Source: CAD feature listing. Evaluate the final solid. Frame: model axes, mm. A direction names the side the tool comes from. Round coordinates to 2 decimals unless told otherwise and drop trailing zeros. Loops run counter-clockwise (first coordinate to the right, second up) from the corner with the lowest first, then second, coordinate; pieces in that order, holes last. Notation, with made-up numbers: (49.25, 89.25) - (88.25, 89.25) arc R9 ccw to (88.25, 99.25) - close; hole circle Ø6 at (76.5, 66.5). An arc over 180 degrees is marked (long way). One line per question, with ' | ' between items. Start each with the question number.
1. Cut plane B-B (y = 0.4). Return loops of the section in (x, z).
2. Cut plane A-A (x = 0). Return loops of the section in (y, z).
3. Ray query, line 1 (Z direction, x = -0.5, y = 1.15); line 2 (X direction, y = 0.9, z = 8.5); line 3 (Z direction, x = -4, y = 0.95). Return the intervals inside material, ascending.
4. Cut plane C-C (z = -8.5). Return loops of the section in (x, y).
5. Access query for faces 1 (the cylindrical face through (3.035, 0.76, 4.051)), 2 (the flat face through (2.75, 1, -8)), 3 (the flat face through (-12, 1, -3.75)), 4 (the flat face through (-2.75, 1, 8)). Directions: +Z, -Z, +X, -X, +Y, -Y. A direction counts if a zero-diameter tool reaches every point of the face in a straight line with its end or side. Return the directions, or none.
6. Pin query (flat end, axial travel): pin 1 (1.4 mm diameter, centred on x = 0, z = -11.21, fed in from -Y); pin 2 (0.8 mm diameter, centred on x = 9, y = 0.5, fed in from +Z). Return the tip coordinate at first contact, or that it passes through.
7. Mould query, pull axis X, two halves, no side actions, for faces 5 (the flat face through (9, 1, 3.75)), 6 (the cylindrical face through (0.06, 0.74, -13.957)), 7 (the cylindrical face through (0.36, 0.76, 12.35)). Classes: pulls with the +X half, pulls with the -X half, needs draft (parallel to the pull), parting line crosses it, or undercut.
```python
from build123d import *

# Parameters (mm, degrees)
SKETCH1_W            = 5.5
SKETCH1_H            = 2
SKETCH1_R            = 1.25
SKETCH1_H_2          = 0.125
SKETCH1_H_3          = 3.25
SKETCH1_H_4          = 7.5
SKETCH1_W_2          = 15.49
SKETCH1_W_3          = 2
SKETCH1_W_4          = 8.01
BOSS_EXTRUDE1_DEPTH  = 1.5
M2_CLEARANCE_HOLE1_D = 2.4
FILLET1_R            = 1


with BuildPart() as part:
    # Sketch1 → Boss-Extrude1 (new body)
    # profile 1 of 16: a face of its own
    with BuildSketch(Plane(origin=(0, 0, 0), x_dir=(1, 0, 0), z_dir=(0, 1, 0))):
        with Locations((0, 8)):
            Rectangle(SKETCH1_W, SKETCH1_H)
    # profile 2 of 16: a face of its own
    with BuildSketch(Plane(origin=(0, 0, 0), x_dir=(1, 0, 0), z_dir=(0, 1, 0))):
        with BuildLine():
            Line((2.75, 9.125), (2.75, 11.2072))
            ThreePointArc((2.75, 11.2072), (0, 13.9572), (-2.75, 11.2072))
            Line((-2.75, 11.2072), (-2.75, 9.125))
            Line((-2.75, 9.125), (2.75, 9.125))
        make_face()
        with Locations((0, 11.2072)):
            Circle(SKETCH1_R, mode=Mode.SUBTRACT)
    # profile 3 of 16: a face of its own
    with BuildSketch(Plane(origin=(0, 0, 0), x_dir=(1, 0, 0), z_dir=(0, 1, 0))):
        with Locations((0, 11.2072)):
            Circle(SKETCH1_R)
    # profile 4 of 16: a face of its own
    with BuildSketch(Plane(origin=(0, 0, 0), x_dir=(1, 0, 0), z_dir=(0, 1, 0))):
        with Locations((0, 9.0625)):
            Rectangle(SKETCH1_W, SKETCH1_H_2)
    # profile 5 of 16: a face of its own
    with BuildSketch(Plane(origin=(0, 0, 0), x_dir=(1, 0, 0), z_dir=(0, 1, 0))):
        with Locations((0, 5.375)):
            Rectangle(SKETCH1_W, SKETCH1_H_3)
    # profile 6 of 16: a face of its own
    with BuildSketch(Plane(origin=(0, 0, 0), x_dir=(1, 0, 0), z_dir=(0, 1, 0))):
        Rectangle(SKETCH1_W, SKETCH1_H_4)
    # profile 7 of 16: a face of its own
    with BuildSketch(Plane(origin=(0, 0, 0), x_dir=(1, 0, 0), z_dir=(0, 1, 0))):
        with Locations((0, -5.375)):
            Rectangle(SKETCH1_W, SKETCH1_H_3)
    # profile 8 of 16: a face of its own
    with BuildSketch(Plane(origin=(0, 0, 0), x_dir=(1, 0, 0), z_dir=(0, 1, 0))):
        with Locations((-10.495, 0)):
            Rectangle(SKETCH1_W_2, SKETCH1_H_4)
    # profile 9 of 16: a face of its own
    with BuildSketch(Plane(origin=(0, 0, 0), x_dir=(1, 0, 0), z_dir=(0, 1, 0))):
        with Locations((-19.24, 0)):
            Rectangle(SKETCH1_W_3, SKETCH1_H_4)
    # profile 10 of 16: a face of its own
    with BuildSketch(Plane(origin=(0, 0, 0), x_dir=(1, 0, 0), z_dir=(0, 1, 0))):
        with Locations((6.755, 0)):
            Rectangle(SKETCH1_W_4, SKETCH1_H_4)
    # profile 11 of 16: a face of its own
    with BuildSketch(Plane(origin=(0, 0, 0), x_dir=(1, 0, 0), z_dir=(0, 1, 0))):
        with Locations((11.76, 0)):
            Rectangle(SKETCH1_W_3, SKETCH1_H_4)
    # profile 12 of 16: a face of its own
    with BuildSketch(Plane(origin=(0, 0, 0), x_dir=(1, 0, 0), z_dir=(0, 1, 0))):
        with Locations((13.76, 0)):
            Rectangle(SKETCH1_W_3, SKETCH1_H_4)
    # profile 13 of 16: a face of its own
    with BuildSketch(Plane(origin=(0, 0, 0), x_dir=(1, 0, 0), z_dir=(0, 1, 0))):
        with Locations((0, -8)):
            Rectangle(SKETCH1_W, SKETCH1_H)
    # profile 14 of 16: a face of its own
    with BuildSketch(Plane(origin=(0, 0, 0), x_dir=(1, 0, 0), z_dir=(0, 1, 0))):
        with BuildLine():
            Line((2.75, -11.2072), (2.75, -9.125))
            Line((2.75, -9.125), (-2.75, -9.125))
            Line((-2.75, -9.125), (-2.75, -11.2072))
            ThreePointArc((-2.75, -11.2072), (0, -13.9572), (2.75, -11.2072))
        make_face()
        with Locations((0, -11.2072)):
            Circle(SKETCH1_R, mode=Mode.SUBTRACT)
    # profile 15 of 16: a face of its own
    with BuildSketch(Plane(origin=(0, 0, 0), x_dir=(1, 0, 0), z_dir=(0, 1, 0))):
        with Locations((0, -11.2072)):
            Circle(SKETCH1_R)
    # profile 16 of 16: a face of its own
    with BuildSketch(Plane(origin=(0, 0, 0), x_dir=(1, 0, 0), z_dir=(0, 1, 0))):
        with Locations((0, -9.0625)):
            Rectangle(SKETCH1_W, SKETCH1_H_2)
    extrude(amount=BOSS_EXTRUDE1_DEPTH)

    # M2 Clearance Hole1 (through all)
    with Locations(Plane(origin=(0, 0, -11.2072), x_dir=(0, 0, -1), z_dir=(0, -1, 0))):
        with Locations((0, 0), (-22.4144, 0)):
            Hole(M2_CLEARANCE_HOLE1_D / 2)

    # Fillet1
    fillet1_edges = [part.edges().sort_by_distance(p)[0] for p in [
        (2.75, 0.75, -3.75),
        (14.76, 0.75, -3.75),
        (14.76, 0.75, 3.75),
        (2.75, 0.75, 3.75),
        (-2.75, 0.75, 3.75),
        (-20.24, 0.75, 3.75),
        (-20.24, 0.75, -3.75),
        (-2.75, 0.75, -3.75),
    ]]
    fillet(fillet1_edges, radius=FILLET1_R)


solid = part.part
```
Answers follow:
1) outline: (-20.24, -2.75) arc R1 ccw to (-19.24, -3.75) - (-3.75, -3.75) arc R1 cw to (-2.75, -4.75) - (-2.75, -11.21) arc R2.75 ccw to (2.75, -11.21) - (2.75, -4.75) arc R1 cw to (3.75, -3.75) - (13.76, -3.75) arc R1 ccw to (14.76, -2.75) - (14.76, 2.75) arc R1 ccw to (13.76, 3.75) - (3.75, 3.75) arc R1 cw to (2.75, 4.75) - (2.75, 11.21) arc R2.75 ccw to (-2.75, 11.21) - (-2.75, 4.75) arc R1 cw to (-3.75, 3.75) - (-19.24, 3.75) arc R1 ccw to (-20.24, 2.75) - close; hole circle Ø2.4 at (0, -11.21); hole circle Ø2.4 at (0, 11.21)
2) outline: (0, -13.96) - (1.5, -13.96) - (1.5, -12.41) - (0, -12.41) - close; (0, -10.01) - (1.5, -10.01) - (1.5, 10.01) - (0, 10.01) - close; (0, 12.41) - (1.5, 12.41) - (1.5, 13.96) - (0, 13.96) - close
3) line 1: z = -13.91 to -12.3, -10.12 to 10.12, 12.3 to 13.91 | line 2: x = -2.75 to 2.75 | line 3: z = -3.75 to 3.75
4) outline: (-2.75, 0) - (2.75, 0) - (2.75, 1.5) - (-2.75, 1.5) - close
5) face 1: +Z, +X, +Y, -Y | face 2: -Z, +X, +Y, -Y | face 3: -Z, -X, +Y, -Y | face 4: +Z, -X, +Y, -Y
6) pin 1: passes through | pin 2: stops at z = 3.75
7) face 5: needs draft | face 6: parting line crosses it | face 7: undercut
